```python
from build123d import *

# Parameters (mm, degrees)
BOSS_EXTRUDE1_DEPTH   = 180
RIB3_REACH            = 124.404
SKETCH4_WALL_W        = 264.810334732
SKETCH4_WALL_H        = 3
RIB4_START            = -3
RIB4_DEPTH            = 3
F_6_CLEARANCE_HOLE1_D = 3.7973
SKETCH6_R             = 2.3495
CUT_EXTRUDE1_DEPTH    = 7
SKETCH12_R            = 2.6162
CUT_EXTRUDE2_DEPTH    = 6.35


# Read off the part's stored shape, not the designer's step: Rib4
with BuildPart() as part:
    # Sketch1 → Boss-Extrude1 (new body)
    with BuildSketch(Plane.XY):
        with BuildLine():
            Line((0, 0), (0, 11.25))
            Line((0, 11.25), (-8, 11.25))
            Line((-8, 11.25), (-8, 6))
            ThreePointArc((-8, 6), (-8.878679656, 3.878679656), (-11, 3))
            Line((-11, 3), (-24, 3))
            Line((-24, 3), (-24, 0))
            Line((-24, 0), (0, 0))
        make_face()
    extrude(amount=BOSS_EXTRUDE1_DEPTH)

    # Sketch4 wall → Rib3 (add, up to next)
    with BuildSketch(Plane(origin=(-16, 7.125, 60.5), x_dir=(-0.888803167408, -0.458289133195, 0), z_dir=(-0.458289133195, 0.888803167408, 0)), mode=Mode.PRIVATE) as rib3_sk1:
        Rectangle(SKETCH4_WALL_W, SKETCH4_WALL_H)
    rib3_tool1 = extrude(rib3_sk1.sketch, amount=-RIB3_REACH, mode=Mode.PRIVATE) - part.part
    rib3 = rib3_tool1.solids().sort_by_distance((-16, 7.125, 60.5))[0]
    add(rib3)

    # Rib4 outline → Rib4 (add)
    with BuildSketch(Plane(origin=(0, 0, 0), x_dir=(-1, 0, 0), z_dir=(0, 0, -1)).offset(RIB4_START)):
        with BuildLine():
            Line((24, 3), (8, 11.25))
            Line((8, 11.25), (8, 6))
            ThreePointArc((8, 6), (8.878679656, 3.878679656), (11, 3))
            Line((11, 3), (24, 3))
        make_face()
    rib4 = extrude(amount=RIB4_DEPTH)

    # Mirror1: Rib3, Rib4 across plane
    add(rib3.mirror(Plane(origin=(0, 0, 90), x_dir=(1, 0, 0), z_dir=(0, 0, -1))))
    add(rib4.mirror(Plane(origin=(0, 0, 90), x_dir=(1, 0, 0), z_dir=(0, 0, -1))))

    # #6 Clearance Hole1 (through all)
    with Locations(Plane(origin=(0, 0, 0), x_dir=(-1, 0, 0), z_dir=(0, -1, 0))):
        with Locations((17.5, -31), (17.5, -149), (17.5, -90)):
            Hole(F_6_CLEARANCE_HOLE1_D / 2)

    # Sketch6 → Cut-Extrude1 (cut)
    with BuildSketch(Plane(origin=(0, 0, 0), x_dir=(0, 0, -1), z_dir=(1, 0, 0))):
        with Locations((-149, 5.625)):
            Circle(SKETCH6_R)
        with Locations((-31, 5.625)):
            Circle(SKETCH6_R)
        with Locations((-90, 5.625)):
            Circle(SKETCH6_R)
    extrude(amount=-CUT_EXTRUDE1_DEPTH, mode=Mode.SUBTRACT)

    # Sketch12 → Cut-Extrude2 (cut)
    with BuildSketch(Plane(origin=(0, 0, 0), x_dir=(0, 0, -1), z_dir=(1, 0, 0))):
        with Locations((-149, 5.625)):
            Circle(SKETCH12_R)
        with Locations((-31, 5.625)):
            Circle(SKETCH12_R)
        with Locations((-90, 5.625)):
            Circle(SKETCH12_R)
    extrude(amount=-CUT_EXTRUDE2_DEPTH, mode=Mode.SUBTRACT)


solid = part.part
```
For this review, take the finished solid that the model builds, in its own axes (mm). A direction names the side the tool comes from. Round coordinates to 2 decimals unless told otherwise and drop trailing zeros. Write each loop counter-clockwise with the first axis right and the second up, starting at its lowest first coordinate (ties: lowest second). Pieces come first, ordered by that corner, then holes. Notation, with made-up numbers: (50, -25.75) -> (109, -25.75) arc R30 ccw to (109, 9.25) -> close; hole circle Ø1 at (-8, 4). An arc over 180 degrees is marked (long way). One line per question, with ' | ' between items. Start each with the question number.
1) For pin 1 Ø4 at (y, z) = (9, 153.5) entering from -X; pin 2 Ø2 at (x, z) = (-21.5, 98) entering from -Y; pin 3 Ø6.5 at (x, z) = (-16, 17.5) entering from +Y; pin 4 Ø3 at (y, z) = (5.625, 31) entering from +X, all flat-tipped, find the tip position at first contact; note any pin that passes through.
2) Add section B-B (x = -17.5). Write out the cut boundary in (y, z), and give its area (3 significant figures).
3) Add section A-A (z = 90). Write out the cut boundary in (x, y).
4) Add section C-C (x = -4.75). Write out the cut boundary in (y, z) (3 decimals).
5) Wall thickness on line 1 along Z through (x, y) = (-15.5, 7); line 2 along Z through (x, y) = (-17.5, 2.1); line 3 along Y through (x, z) = (-4.25, 31): over which ranges is each line inside the solid? List them lowest first.
6) Add section D-D (z = 154). Write out the cut boundary in (x, y), and give its area (3 significant figures).
7) Machinability: for faces 1 (the flat face through (-13, 6, 62)), 2 (the cylindrical face through (-6.67, 4.725, 146.83)), 3 (the flat face through (-4, 11.25, 89)), which of the approach directions +Z, -Z, +X, -X, +Y, -Y give a long, thin tool a straight path to every point of the face, cutting with its end or side? Answer none if there is none.
8) Mouldability with a two-part tool opening along Z and no side actions: class faces 4 (the flat face through (-16.11, 7.07, 178.48)), 5 (the flat face through (-8, 9, 31)) as +Z half, -Z half, draft (parallel to the pull), parting line (faces both ways), or undercut.
Reported:
1) pin 1: stops at x = -8 | pin 2: stops at y = 0 | pin 3: stops at y = 3 | pin 4: stops at x = -7
2) outline: (0, 0) -> (6.35, 0) -> (6.35, 3) -> (3, 3) -> (3, 29.1) -> (0, 29.1) -> close; (0, 32.9) -> (3, 32.9) -> (3, 59) -> (6.35, 59) -> (6.35, 62) -> (3, 62) -> (3, 88.1) -> (0, 88.1) -> close; (0, 91.9) -> (3, 91.9) -> (3, 118) -> (6.35, 118) -> (6.35, 121) -> (3, 121) -> (3, 147.1) -> (0, 147.1) -> close; (0, 150.9) -> (3, 150.9) -> (3, 177) -> (6.35, 177) -> (6.35, 180) -> (0, 180) -> close | area: 546 mm²
3) outline: (-24, 0) -> (-19.4, 0) -> (-19.4, 3) -> (-24, 3) -> close; (-15.6, 0) -> (0, 0) -> (0, 3.01) -> (-6.35, 3.01) -> (-6.35, 3.28) -> (-7, 3.28) -> (-7, 7.97) -> (-6.35, 7.97) -> (-6.35, 8.24) -> (0, 8.24) -> (0, 11.25) -> (-8, 11.25) -> (-8, 6) arc R3 cw to (-11, 3) -> (-15.6, 3) -> close
4) outline: (0, 0) -> (11.25, 0) -> (11.25, 180) -> (0, 180) -> close; hole circle Ø5.232 at (5.625, 31); hole circle Ø5.232 at (5.625, 90); hole circle Ø5.232 at (5.625, 149)
5) line 1: z = 0 to 3, 59 to 62, 118 to 121, 177 to 180 | line 2: z = 0 to 29.1, 32.9 to 88.1, 91.9 to 147.1, 150.9 to 180 | line 3: y = 0 to 3.01, 8.24 to 11.25
6) outline: (-24, 0) -> (0, 0) -> (0, 11.25) -> (-8, 11.25) -> (-8, 6) arc R3 cw to (-11, 3) -> (-24, 3) -> close | area: 140 mm²
7) face 1: -X, +Y | face 2: +X | face 3: +Z, -Z, +X, -X, +Y
8) face 4: draft | face 5: undercut
